The model under review builds one solid part; all positions refer to its coordinate system, in mm. Give positions to 0.01 mm unless a question says otherwise; leave off trailing zeros. Loops run counter-clockwise (first coordinate to the right, second up) from the corner with the lowest first, then second, coordinate; pieces in that order, holes last. Notation, with made-up numbers: M 88,77 L 131,77 A14 ccw 131,89 Z; hole C 22,-15.75 d5. An arc over 180 degrees is marked long. One line per item, written item: value. Start each with the question number.
Q1. To check wall thickness, follow line 1 along X through (y, z) = (45, 3); line 2 along Y through (x, z) = (1, 2); line 3 along Y through (x, z) = (-5, 0.5). State the ranges of each line that lie inside material, in increasing order. Write a range as from..to.
Q2. We need section C-C on x = -10. Write out the cut boundary in (y, z).
Q3. For pin 1 (8 mm diameter, centred on x = 8, y = 14.5, fed in from -Z); pin 2 (4 mm diameter, centred on y = 50.5, z = 4, fed in from +X), all flat-tipped, find the tip position at first contact; note any pin that passes through.
Q4. We need section A-A on y = 38.5. Write out the cut boundary in (x, z).
Q5. We need section D-D on y = 9. Write out the cut boundary in (x, z).
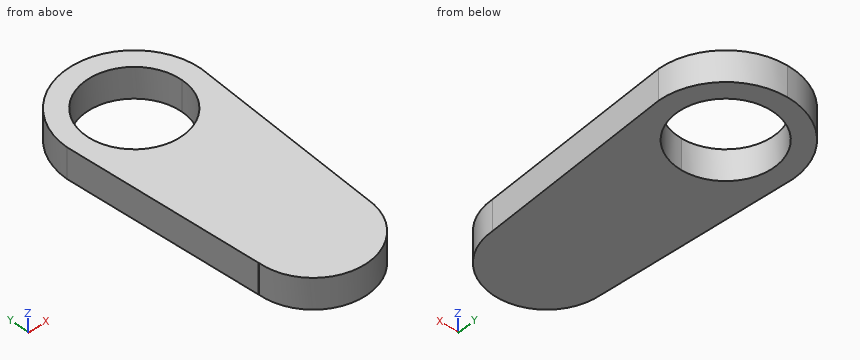
```python
from build123d import *

# Parameters (mm, degrees)
F1_DEPTH = 7


with BuildPart() as f1:
    # F0 (on Top) → F1 (new body)
    with BuildSketch(Plane.XY):
        with BuildLine():
            Line((0, 0), (12.6, 0))
            ThreePointArc((12.6, 0), (8.909545443, 8.909545443), (0, 12.6))
            Line((0, 12.6), (0, 0))
        make_face()
        with BuildLine():
            ThreePointArc((-12.6, 0), (0, -12.6), (12.6, 0))
            Line((12.6, 0), (0, 0))
            Line((0, 0), (-12.6, 0))
        make_face()
        with BuildLine():
            ThreePointArc((0, 12.6), (8.909545443, 8.909545443), (12.6, 0))
            Line((12.6, 0), (15.5728551745, 45))
            ThreePointArc((15.5728551745, 45), (11.0116714964, 56.0116714964), (0, 60.5728551745))
            ThreePointArc((0, 60.5728551745), (-11.0116714964, 56.0116714964), (-15.5728551745, 45))
            Line((-15.5728551745, 45), (-12.6269701008, 0))
            Line((-12.6269701008, 0), (-12.6, 0))
            ThreePointArc((-12.6, 0), (-8.909545443, 8.909545443), (0, 12.6))
        make_face()
        with BuildLine():
            ThreePointArc((11.1, 45), (7.8488852712, 37.1511147288), (0, 33.9))
            ThreePointArc((0, 33.9), (-7.8488852712, 52.8488852712), (11.1, 45))
        make_face(mode=Mode.SUBTRACT)
        with BuildLine():
            Line((0, 0), (0, 12.6))
            ThreePointArc((0, 12.6), (-8.909545443, 8.909545443), (-12.6, 0))
            Line((-12.6, 0), (0, 0))
        make_face()
    extrude(amount=F1_DEPTH)


solid = f1.part
```
Solved:
1. line 1: -15.57..-11.1, 11.1..15.57
1. line 2: -12.56..33.95, 56.05..60.54
1. line 3: -11.57..35.09, 54.91..59.75
2. outline: M -7.67,0 L 40.18,0 L 40.18,7 L -7.67,7 Z; M 49.82,0 L 56.94,0 L 56.94,7 L 49.82,7 Z
3. pin 1: z = 0
3. pin 2: x = 15.17
4. outline: M -15.15,0 L -9,0 L -9,7 L -15.15,7 Z; M 9,0 L 15.14,0 L 15.14,7 L 9,7 Z
5. outline: M -13.22,0 L 13.19,0 L 13.19,7 L -13.22,7 Z
